Geometry check sheet. Reference: drawing and pictorial views, mm from the part's lowest x, y, z. Round coordinates to 2 decimals unless told otherwise and drop trailing zeros. Order: outer loops, then holes, each group sorted by start corner. A loop starts at its lowest first (then second) coordinate and runs counter-clockwise, first axis right, second up.
Q1. Depth check by flat-ended pin: P1, Ø13, axis at y = 544, z = 31.5, coming from the -X side; P2, Ø9.5, axis at y = 5, z = 85.5, coming from the -X side; P3, Ø6, axis at x = 8, y = 406, coming from the +Z side; P4, Ø9, axis at y = 449.5, z = 144, coming from the -X side. Enter the tip coordinate at first touch or a pass-through.
Q2. Scan lines: probe 1 along Z at (x, y) = (7.25, 90); probe 2 along Y at (x, z) = (1.75, 88.5); probe 3 along Z at (x, y) = (10, 139). Record each from-to range of solid material in increasing order.
Q3. Cross-section at A-A on y = 102.5. Record the cut outline in (x, z).
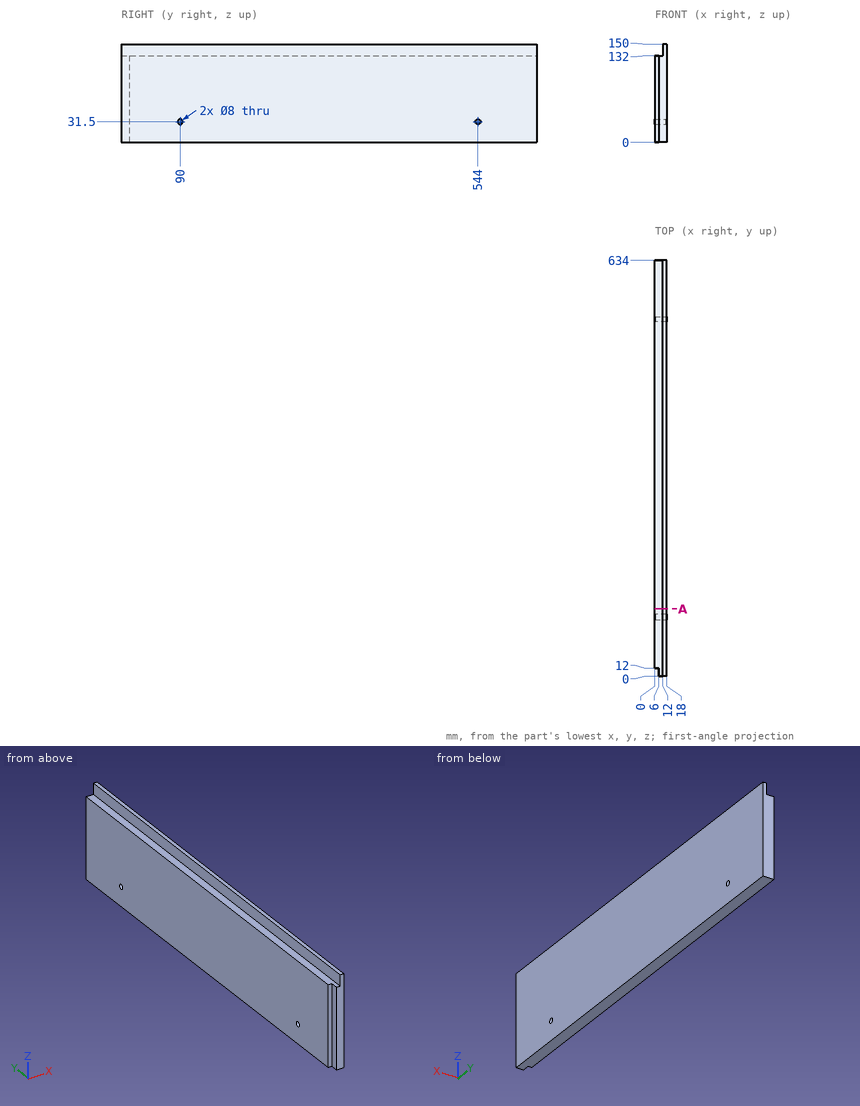
Results found:
1. P1: stops at x = 0
1. P2: stops at x = 6
1. P3: stops at z = 132
1. P4: stops at x = 12
2. probe 1: z = 0 to 27.5, 35.5 to 132
2. probe 2: y = 12 to 634
2. probe 3: z = 0 to 132
3. outline: (0, 0) - (18, 0) - (18, 150) - (12, 150) - (12, 132) - (0, 132) - close
